Autodesk Inventor part; units mm, degrees
ref_plane "YZ Plane" through (0, 0, 0) normal (1, 0, 0) x (0, 1, 0)
ref_plane "XZ Plane" through (0, 0, 0) normal (0, 1, 0) x (-1, 0, 0)
ref_plane "XY Plane" through (0, 0, 0) normal (0, 0, 1) x (1, 0, 0)
ref_plane "Work Plane5" through (0, 0, 10) normal (0, 0, 1) x (1, 0, 0)
sketch "Sketch1" plane through (0, 0, 10) normal (0, 0, 1) x (1, 0, 0)
  line L0 (-4.0299, -0.3538) -> (-2.2322, 1.4439) construction
  arc A0 (-1.4439, 2.2322) -> (-2.2322, 1.4439) centre (-0.9299, 0.9299) ccw construction
  line L1 (-1.4439, 2.2322) -> (0.3538, 4.0299) construction
  line L2 (-37.8299, 42.8299) -> (-37.8299, 37.8299) construction
  line L3 (-37.8299, 37.8299) -> (-42.9208, 37.8299) construction
  line L4 (-37.8299, 42.2137) -> (-37.8299, 45.8299) construction
  line L5 (-37.8299, 45.8299) -> (-4.0299, 45.8299) construction
  line L6 (-4.0299, 45.8299) -> (-4.0299, 42.2137) construction
  line L7 (-4.0299, 4.0299) -> (0.3538, 4.0299)
  circle A1 centre (-20.9299, 20.9299) radius 17.5
  line L8 (-20.9299, 58.9723) -> (17.1124, 20.9299) construction
  line L9 (17.1124, 20.9299) -> (-20.9299, -17.1124) construction
  line L10 (-20.9299, -17.1124) -> (-58.9723, 20.9299) construction
  line L11 (-58.9723, 20.9299) -> (-20.9299, 58.9723) construction
  line L12 (-20.9299, 58.9723) -> (-20.9299, -17.1124) construction
  line L13 (17.1124, 20.9299) -> (-58.9723, 20.9299) construction
  line L14 (-20.9299, 58.9723) -> (32.8701, 58.9723) construction
  line L15 (-43.4299, 43.4299) -> (1.5701, 43.4299) construction
  line L16 (1.5701, 43.4299) -> (1.5701, -1.5701) construction
  line L17 (1.5701, -1.5701) -> (-43.4299, -1.5701) construction
  line L18 (-43.4299, -1.5701) -> (-43.4299, 43.4299) construction
  line L19 (-43.4299, 43.4299) -> (1.5701, -1.5701) construction
  line L20 (1.5701, 43.4299) -> (-43.4299, -1.5701) construction
  line L21 (-43.4299, 5.3876) -> (-43.4299, 36.4723)
  line L22 (-43.4299, 36.4723) -> (-36.4723, 43.4299)
  line L23 (-36.4723, 43.4299) -> (-5.3876, 43.4299)
  line L24 (-5.3876, 43.4299) -> (1.5701, 36.4723)
  line L25 (1.5701, 36.4723) -> (1.5701, 5.3876)
  line L26 (1.5701, 5.3876) -> (-5.3876, -1.5701)
  line L27 (-5.3876, -1.5701) -> (-36.4723, -1.5701)
  line L28 (-36.4723, -1.5701) -> (-43.4299, 5.3876)
  line L29 (-4.0299, 42.2137) -> (-37.8299, 42.2137)
  line L30 (-4.0299, -0.3538) -> (-4.0299, 4.0299)
  circle A2 centre (-20.9299, 20.9299) radius 1.5
  line L31 (-10.9299, 10.9299) -> (-30.9299, 10.9299) construction
  line L32 (-30.9299, 10.9299) -> (-30.9299, 30.9299) construction
  line L33 (-30.9299, 30.9299) -> (-10.9299, 30.9299) construction
  line L34 (-10.9299, 30.9299) -> (-10.9299, 10.9299) construction
  line L35 (-10.9299, 10.9299) -> (-30.9299, 30.9299) construction
  line L36 (-30.9299, 10.9299) -> (-10.9299, 30.9299) construction
  circle A3 centre (-30.9299, 30.9299) radius 1.4
  circle A4 centre (-30.9299, 10.9299) radius 1.4
  circle A5 centre (-10.9299, 10.9299) radius 1.4
  line L37 (-45.8299, 37.8299) -> (-42.0723, 37.8299) construction
  line L38 (-42.1723, 37.7299) -> (-45.8299, 37.7299)
  line L39 (-45.8299, 37.7299) -> (-45.8299, 4.1299)
  line L40 (-45.8299, 4.1299) -> (-42.1723, 4.1299)
  line L41 (-42.1723, 4.1299) -> (-42.1723, 37.7299)
  line L42 (-45.8299, 4.0299) -> (-42.0723, 4.0299) construction
  line L43 (-45.8299, 37.8299) -> (-42.0723, 37.8299)
  line L44 (-37.7299, 45.8299) -> (-4.1299, 45.8299)
  line L45 (-4.1299, 45.8299) -> (-4.1299, 42.1723)
  line L46 (-4.1299, 42.1723) -> (-37.7299, 42.1723)
  line L47 (-37.7299, 42.1723) -> (-37.7299, 45.8299)
  line L48 (0.4701, 37.8299) -> (0.4701, 4.0299) construction
  line L49 (0.4701, 4.0299) -> (3.9701, 4.0299) construction
  line L50 (3.9701, 37.8299) -> (3.9701, 4.0299) construction
  line L51 (0.4701, 37.8299) -> (3.9701, 37.8299) construction
  line L52 (-45.8299, -3.9701) -> (-4.0299, -3.9701) construction
  line L53 (0.3124, 37.7299) -> (3.9701, 37.7299)
  line L54 (3.9701, 37.7299) -> (3.9701, 4.1299)
  line L55 (3.9701, 4.1299) -> (0.3124, 4.1299)
  line L56 (0.3124, 4.1299) -> (0.3124, 37.7299)
  line L57 (-4.1713, -0.3538) -> (-37.7299, -0.3538)
  line L58 (-37.7299, -0.3538) -> (-37.7299, -3.9701)
  line L59 (-37.7299, -3.9701) -> (-4.1713, -3.9701)
  line L60 (-4.1713, -3.9701) -> (-4.1713, -0.3538)
  point P0 (-37.8299, 4.0299)
  dimension "d18" = 53.8
  dimension "d19" = 45
  dimension "d20" = 53.8
  dimension "d21" = 45
  dimension "d22" = 45
  dimension "d30" = 20
  dimension "d31" = 20
  dimension "d32" = 2.8
  dimension "d33" = 2.8
  dimension "d34" = 2.8
  dimension "d35" = 3
  dimension "d36" = 0.1
  dimension "d37" = 0.1
  dimension "d38" = 0.1
  dimension "d39" = 0.1
extrude "Extrusion1" add sketch "Sketch1" along normal blind 10 contours L30 L26 L57 L28 L41 L22 L46 L24 L56 L7 | L7 L26 L30 | L56 L24 L25 L26 | L26 L25 L24 L53 L54 L55 | L60 L59 L58 L57 L28 L27 L26 | L26 L27 L28 L57 | L46 L22 L29 L24 | L24 L29 L45 | L40 L39 L38 L22 L21 L28 | L28 L21 L22 L41 | L29 L22 L23 L24 | L24 L23 L22 L29 L47 L44 L45 | L47 L29 L22 | A1 | A2 | A3 | A4 | A5
sketch "Skizze4" plane through (0, 0, 20) normal (0, 0, 1) x (1, 0, 0)
  line L0 (-37.7299, 42.1723) -> (-42.1723, 37.7299)
  line L1 (-42.1723, 37.7299) -> (-45.8299, 37.7299)
  line L2 (-45.8299, 37.7299) -> (-45.8299, 4.1299) construction
  line L3 (-45.8299, 4.1299) -> (-42.1723, 4.1299)
  line L4 (-42.1723, 4.1299) -> (-37.6885, -0.3538)
  line L5 (-37.6885, -0.3538) -> (-37.7299, -0.3538)
  line L6 (-37.7299, -0.3538) -> (-37.7299, -3.9701)
  line L7 (-37.7299, -3.9701) -> (-4.1713, -3.9701) construction
  line L8 (-4.1713, -3.9701) -> (-4.1713, -0.3538)
  line L9 (-4.1713, -0.3538) -> (0.3124, 4.1299)
  line L10 (0.3124, 4.1299) -> (3.9701, 4.1299)
  line L11 (3.9701, 4.1299) -> (3.9701, 37.7299) construction
  line L12 (3.9701, 37.7299) -> (0.3124, 37.7299)
  line L13 (0.3124, 37.7299) -> (-4.1299, 42.1723)
  line L14 (-4.1299, 42.1723) -> (-4.1299, 45.8299)
  line L15 (-4.1299, 45.8299) -> (-37.7299, 45.8299) construction
  line L16 (-37.7299, 45.8299) -> (-37.7299, 42.1723)
  line L17 (-37.9299, 46.0299) -> (-3.9299, 46.0299) construction
  line L18 (-3.9299, 46.0299) -> (-3.9299, 42.2551)
  line L19 (-3.9299, 42.2551) -> (0.3953, 37.9299)
  line L20 (0.3953, 37.9299) -> (4.1701, 37.9299)
  line L21 (4.1701, 37.9299) -> (4.1701, 3.9299) construction
  line L22 (4.1701, 3.9299) -> (0.3953, 3.9299)
  line L23 (0.3953, 3.9299) -> (-3.9713, -0.4367)
  line L24 (-3.9713, -0.4367) -> (-3.9713, -4.1701)
  line L25 (-3.9713, -4.1701) -> (-37.9299, -4.1701) construction
  line L26 (-37.9299, -4.1701) -> (-37.9299, -0.3953)
  line L27 (-37.9299, -0.3953) -> (-42.2551, 3.9299)
  line L28 (-42.2551, 3.9299) -> (-46.0299, 3.9299)
  line L29 (-46.0299, 3.9299) -> (-46.0299, 37.9299) construction
  line L30 (-46.0299, 37.9299) -> (-42.2551, 37.9299)
  line L31 (-42.2551, 37.9299) -> (-37.9299, 42.2551)
  line L32 (-37.9299, 42.2551) -> (-37.9299, 46.0299)
  line L33 (-45.8299, 37.7299) -> (-45.8299, 37.9299)
  line L34 (-4.1299, 45.8299) -> (-37.7299, 45.8299)
  line L35 (-37.7299, 45.8299) -> (-37.9299, 45.8299)
  line L36 (-4.1299, 45.8299) -> (-3.9299, 45.8299)
  line L37 (3.9701, 37.7299) -> (3.9701, 37.9299)
  line L38 (3.9701, 4.1299) -> (3.9701, 37.7299)
  line L39 (3.9701, 4.1299) -> (3.9701, 3.9299)
  line L40 (-4.1713, -3.9701) -> (-3.9713, -3.9701)
  line L41 (-37.7299, -3.9701) -> (-37.9299, -3.9701)
  line L42 (-45.8299, 4.1299) -> (-45.8299, 3.9299)
  point P0 (0, 0)
  dimension "d40" = 0.2
extrude "IM_offset" add sketch "Skizze4" against normal up to surface (10 mm away)
sketch "Sketch29" plane through (0, 0, 10) normal (0, 0, -1) x (-1, 0, 0)
  arc A0 (32.4799, 17.9099) -> (35.0799, 20.5099) centre (32.4799, 20.5099) ccw
  arc A1 (9.4799, 46.1099) -> (6.8799, 43.5099) centre (9.4799, 43.5099) ccw
  arc A2 (35.0799, 43.5099) -> (32.4799, 46.1099) centre (32.4799, 43.5099) ccw
  arc A3 (6.8799, 20.5099) -> (9.4799, 17.9099) centre (9.4799, 20.5099) ccw
  line L0 (35.0799, 17.9099) -> (6.8799, 17.9099)
  line L1 (6.8799, 17.9099) -> (6.8799, 46.516)
  line L2 (6.8799, 46.516) -> (35.0799, 46.516)
  line L3 (35.0799, 46.516) -> (35.0799, 17.9099)
  line L4 (35.2799, 17.7099) -> (6.6799, 17.7099)
  line L5 (6.6799, 17.7099) -> (6.6799, 46.716)
  line L6 (6.6799, 46.716) -> (35.2799, 46.716)
  line L7 (35.2799, 46.716) -> (35.2799, 17.7099)
  point P0 (0, 0)
  point P1 (6.8799, 20.5099)
  point P2 (9.4799, 17.9099)
  point P3 (32.4799, 17.9099)
  point P4 (35.0799, 20.5099)
  dimension "d171" = 0.2
extrude "Extrusion23" cut sketch "Sketch29" against normal blind 10 contours L0 A3 L1 L2 L3 A0
sketch "Sketch30" plane through (0, 0, 10) normal (0, 0, -1) x (-1, 0, 0)
  line L0 (35.0799, 45.8299) -> (35.0799, 20.5099)
  arc A0 (32.4799, 17.9099) -> (35.0799, 20.5099) centre (32.4799, 20.5099) ccw
  line L1 (32.4799, 17.9099) -> (9.4799, 17.9099)
  arc A1 (6.8799, 20.5099) -> (9.4799, 17.9099) centre (9.4799, 20.5099) ccw
  line L2 (6.8799, 20.5099) -> (6.8799, 45.8299)
  line L3 (6.8799, 45.8299) -> (3.9299, 45.8299)
  line L4 (3.9299, 45.8299) -> (3.9299, 42.2551)
  line L5 (3.9299, 42.2551) -> (-0.3953, 37.9299)
  line L6 (-0.3953, 37.9299) -> (-3.9701, 37.9299)
  line L7 (-3.9701, 37.9299) -> (-3.9701, 3.9299)
  line L8 (-3.9701, 3.9299) -> (-0.3953, 3.9299)
  line L9 (-0.3953, 3.9299) -> (3.9713, -0.4367)
  line L10 (3.9713, -0.4367) -> (3.9713, -3.9701)
  line L11 (3.9713, -3.9701) -> (37.9299, -3.9701)
  line L12 (37.9299, -3.9701) -> (37.9299, -0.3953)
  line L13 (37.9299, -0.3953) -> (42.2551, 3.9299)
  line L14 (42.2551, 3.9299) -> (45.8299, 3.9299)
  line L15 (45.8299, 3.9299) -> (45.8299, 37.9299)
  line L16 (45.8299, 37.9299) -> (42.2551, 37.9299)
  line L17 (42.2551, 37.9299) -> (37.9299, 42.2551)
  line L18 (37.9299, 42.2551) -> (37.9299, 45.8299)
  line L19 (37.9299, 45.8299) -> (35.0799, 45.8299)
  line L20 (37.9299, 45.8299) -> (35.0799, 45.8299)
  line L21 (6.8799, 20.5099) -> (6.8799, 45.8299)
  line L22 (35.0799, 45.8299) -> (6.8799, 45.8299)
  point P0 (0, 0)
extrude "Extrusion24" add sketch "Sketch30" against normal blind 0.5 contours L0 A0 L1 A1 L2 L22
ref_plane "Arbeitsebene7" through (-20.9299, 3.9299, 10) normal (-1, 0, 0) x (0, 0, 1)
ref_plane "Arbeitsebene8" through (-37.9299, 20.9299, 10) normal (0, 1, 0) x (1, 0, 0)
ref_plane "Arbeitsebene9" through (-20.9299, 3.9299, 10) normal (-1, 0, 0) x (0, 0, 1)
ref_plane "Arbeitsebene10" through (-37.9299, 20.9299, 10) normal (0, -1, 0) x (1, 0, 0)
properties part number "20_Cube_Insert_Fiber_STMount_Center"
For this review, take the finished solid that the model builds, in its own axes (mm). A direction names the side the tool comes from. Round coordinates to 2 decimals unless told otherwise and drop trailing zeros. Loops run counter-clockwise (first coordinate to the right, second up) from the corner with the lowest first, then second, coordinate; pieces in that order, holes last.
Q1. Add section A-A on y = 21.5. Write out the cut boundary in (x, z).
Result sheet:
outline: (-45.83, 10) - (3.97, 10) - (3.97, 20) - (-6.88, 20) - (-6.88, 10.5) - (-35.08, 10.5) - (-35.08, 20) - (-45.83, 20) - close
Q2. Add section D-D on y = 41.5. Write out the cut boundary in (x, z) (3 decimals).
Result sheet:
outline: (-38.685, 10) - (-3.175, 10) - (-3.175, 20) - (-6.88, 20) - (-6.88, 10.5) - (-35.08, 10.5) - (-35.08, 20) - (-38.685, 20) - close
Q3. Insertion check: pin 1 Ø3 at (y, z) = (-3, 14) entering from +X; pin 2 Ø3 at (y, z) = (45, 13.5) entering from -X; pin 3 Ø1.8 at (x, z) = (-45, 16) entering from -Y. Each pin has a flat end and moves straight along its axis. Give the tip position at first contact, or say it passes through.
Result sheet:
pin 1: stops at x = -3.97
pin 2: stops at x = -37.93
pin 3: stops at y = 3.93
Q4. Machinability: for faces 1 (the face through (-3.971, -2, 15)), 2 (the face through (2, 37.93, 15)), 3 (the face through (-6.88, 33, 15)), 4 (the face through (-44, 3.93, 15)), which of the approach directions +Z, -Z, +X, -X, +Y, -Y give a long, thin tool a straight path to every point of the face, cutting with its end or side? Answer none if there is none.
Result sheet:
face 1: +Z, -Z, +X, -Y
face 2: +Z, -Z, +X, +Y
face 3: +Z, +Y
face 4: +Z, -Z, -X, -Y
Q5. Add section C-C on x = -16.5. Write out the cut boundary in (y, z).
Result sheet:
outline: (-3.97, 10) - (45.83, 10) - (45.83, 10.5) - (17.91, 10.5) - (17.91, 20) - (-3.97, 20) - close
Q6. Add section B-B on z = 16.75. Write out the cut boundary in (x, y), plus the area to 3 significant figures.
Result sheet:
outline: (-45.83, 3.93) - (-42.26, 3.93) - (-37.93, -0.4) - (-37.93, -3.97) - (-3.97, -3.97) - (-3.97, -0.44) - (0.4, 3.93) - (3.97, 3.93) - (3.97, 37.93) - (0.4, 37.93) - (-3.93, 42.26) - (-3.93, 45.83) - (-6.88, 45.83) - (-6.88, 20.51) arc R2.6 cw to (-9.48, 17.91) - (-32.48, 17.91) arc R2.6 cw to (-35.08, 20.51) - (-35.08, 45.83) - (-37.93, 45.83) - (-37.93, 42.26) - (-42.26, 37.93) - (-45.83, 37.93) - close
area: 1,480 mm2
Q7. Mouldability with a two-part tool opening along X and no side actions: class faces 5 (the face through (-21, -3.97, 15)), 6 (the face through (-35.08, 33, 15)), 7 (the face through (-40.062, 1.737, 15.07)) as +X half, -X half, draft (parallel to the pull), parting line (faces both ways), or undercut.
Result sheet:
face 5: draft
face 6: undercut
face 7: -X half
Q8. To check wall thickness, follow line 1 along X through (y, z) = (34.5, 17); line 2 along Y through (x, z) = (-15, 10.75); line 3 along X through (y, z) = (42.5, 11.5). State the ranges of each line that lie inside material, in increasing order.
Result sheet:
line 1: x = -45.83 to -35.08, -6.88 to 3.97
line 2: y = -3.97 to 17.91
line 3: x = -37.93 to -35.08, -6.88 to -3.93
